Source: CAD feature listing. Evaluate the final solid. Frame: model axes, mm. A direction names the side the tool comes from. Give positions to 0.01 mm unless a question says otherwise; leave off trailing zeros. Order: outer loops, then holes, each group sorted by start corner. A loop starts at its lowest first (then second) coordinate and runs counter-clockwise, first axis right, second up. Notation, with made-up numbers: M -22,52 L 22,52 A25 cw 22,75 Z; hole C 54,-16.5 d10. An arc over 180 degrees is marked long. Return JSON: item names as keys, results as strings.
from build123d import *

# Parameters (mm, degrees)
SKETCH2_W           = 12.2
SKETCH2_H           = 11.7
SKETCH2_W_2         = 6.2
SKETCH2_H_2         = 5.7
BOSS_EXTRUDE1_DEPTH = 0.8
SKETCH3_W           = 12.2
SKETCH3_H           = 11.7
SKETCH3_W_2         = 8.5
SKETCH3_H_2         = 8.5
BOSS_EXTRUDE2_DEPTH = 4
SKETCH4_W           = 12.2
SKETCH4_H           = 11.7
SKETCH4_R           = 2.65
BOSS_EXTRUDE3_DEPTH = 4
SKETCH5_W           = 2.5
SKETCH5_H           = 2.5
BOSS_EXTRUDE4_DEPTH = 6.22
SKETCH8_W           = 8.5
SKETCH8_H           = 4
CUT_EXTRUDE2_DEPTH  = 6.22
CUT_EXTRUDE3_DEPTH  = 2


with BuildPart() as part:
    # Sketch2 → Boss-Extrude1 (new body)
    with BuildSketch(Plane(origin=(0, 0, 0), x_dir=(1, 0, 0), z_dir=(0, 1, 0))):
        Rectangle(SKETCH2_W, SKETCH2_H)
        Rectangle(SKETCH2_W_2, SKETCH2_H_2, mode=Mode.SUBTRACT)
    extrude(amount=-BOSS_EXTRUDE1_DEPTH)

    # Sketch3 → Boss-Extrude2 (add)
    with BuildSketch(Plane.XZ.offset(0.8)):
        Rectangle(SKETCH3_W, SKETCH3_H)
        Rectangle(SKETCH3_W_2, SKETCH3_H_2, mode=Mode.SUBTRACT)
    extrude(amount=BOSS_EXTRUDE2_DEPTH)

    # Sketch4 → Boss-Extrude3 (add)
    with BuildSketch(Plane.XZ.offset(4.8)):
        Rectangle(SKETCH4_W, SKETCH4_H)
        with Locations(Location((0, 0, 0), (0, 0, 270))):
            Circle(SKETCH4_R, mode=Mode.SUBTRACT)
    extrude(amount=BOSS_EXTRUDE3_DEPTH)

    # Sketch5 → Boss-Extrude4 (add)
    with BuildSketch(Plane.XZ.offset(8.8)):
        with Locations((-4.85, -4.6)):
            Rectangle(SKETCH5_W, SKETCH5_H)
    extrude(amount=BOSS_EXTRUDE4_DEPTH)

    # Sketch8 → Cut-Extrude2 (cut)
    with BuildSketch(Plane.ZY.offset(-4.25)):
        with Locations((0, -2.8)):
            Rectangle(SKETCH8_W, SKETCH8_H)
    extrude(amount=-CUT_EXTRUDE2_DEPTH, mode=Mode.SUBTRACT)

    # Sketch9 → Cut-Extrude3 (cut)
    with BuildSketch(Plane(origin=(0, 0, 0), x_dir=(1, 0, 0), z_dir=(0, 1, 0))):
        with BuildLine():
            Line((3.1, 2.85), (3.1, -2.85))
            add(Edge.make_bspline(
                [(3.1, 2.85), (3.9, 0), (3.1, -2.85)],
                knots=[0, 0, 0, 1, 1, 1], degree=2))
        make_face()
    extrude(amount=-CUT_EXTRUDE3_DEPTH, mode=Mode.SUBTRACT)


solid = part.part
1. Section query A-A (x = 0). Return loops of the section in (y, z).
Evaluation:
{"outline": "M -8.8,-5.85 L 0,-5.85 L 0,-2.85 L -0.8,-2.85 L -0.8,-4.25 L -4.8,-4.25 L -4.8,-2.65 L -8.8,-2.65 Z; M -8.8,2.65 L -4.8,2.65 L -4.8,4.25 L -0.8,4.25 L -0.8,2.85 L 0,2.85 L 0,5.85 L -8.8,5.85 Z"}
2. Ray query, probe 1 along Y at (x, z) = (-3, 4); probe 2 along X at (y, z) = (-6.75, 0); probe 3 along Z at (x, y) = (-0.25, -4.5). Return the intervals inside material, ascending.
Evaluation:
{"probe 1": "y = -8.8 to -4.8, -0.8 to 0", "probe 2": "x = -6.1 to -2.65, 2.65 to 6.1", "probe 3": "z = -5.85 to -4.25, 4.25 to 5.85"}
3. Section query D-D (x = 4). Return loops of the section in (y, z), then the cut area to 3 significant figures.
Evaluation:
{"outline": "M -8.8,-5.85 L 0,-5.85 L 0,5.85 L -8.8,5.85 Z; hole M -4.8,-4.25 L -0.8,-4.25 L -0.8,4.25 L -4.8,4.25 Z", "area": "69.0 mm^2"}
4. First-contact query: pin 1 (1.2 mm diameter, centred on y = -2.5, z = -0.5, fed in from +X); pin 2 (3 mm diameter, centred on x = -3, y = -10.5, fed in from +Z); pin 3 (3 mm diameter, centred on x = 2, z = 4.5, fed in from -Y); pin 4 (5 mm diameter, centred on x = 0, z = 0, fed in from +Y). Flat tips, straight axial feed; report the tip coordinate or a pass-through.
Evaluation:
{"pin 1": "stops at x = -4.25", "pin 2": "stops at z = -3.35", "pin 3": "stops at y = -8.8", "pin 4": "passes through"}
5. Section query C-C (y = -7.75). Return loops of the section in (x, z), then the cut area to 3 significant figures.
Evaluation:
{"outline": "M -6.1,-5.85 L 6.1,-5.85 L 6.1,5.85 L -6.1,5.85 Z; hole C 0,0 d5.3", "area": "121 mm^2"}
6. Set-up query: faces 1 (the face through (0, -4, 5.85)), 2 (the face through (-4.25, -3, 0)), 3 (the face through (-3.6, -12, -5)). Return all of +Z, -Z, +X, -X, +Y, -Y with unobstructed straight access to the full face (end or side cutting, diameter ignored); none if empty.
Evaluation:
{"face 1": "+Z, +X, -X, +Y, -Y", "face 2": "+X", "face 3": "+Z, -Z, +X, -Y"}
7. Section query B-B (z = 3.5). Return loops of the section in (x, y).
Evaluation:
{"outline": "M -6.1,-8.8 L 6.1,-8.8 L 6.1,-4.8 L -4.25,-4.8 L -4.25,-0.8 L 6.1,-0.8 L 6.1,0 L -6.1,0 Z"}
8. Draft query along Y for faces 4 (the face through (4, -0.8, 0)), 5 (the face through (-5, -15.02, -5)), 6 (the face through (-5, -12, -3.35)). Return one class per face: pulls with the +Y half, pulls with the -Y half, needs draft (parallel to the pull), parting line crosses it, or undercut.
Evaluation:
{"face 4": "undercut", "face 5": "pulls with the -Y half", "face 6": "needs draft"}
